from build123d import *

# Parameters (mm, degrees)
BOSS_EXTRUDE1_DEPTH   = 6
SKETCH2_W             = 71
SKETCH2_H             = 6
BOSS_EXTRUDE2_DEPTH   = 6
CUT_EXTRUDE1_DEPTH    = 6
SKETCH5_W             = 30
SKETCH5_H             = 6
BOSS_EXTRUDE3_DEPTH   = 6
BOSS_EXTRUDE3_2_DEPTH = 6
BOSS_EXTRUDE3_3_DEPTH = 6
BOSS_EXTRUDE3_4_DEPTH = 6


with BuildPart() as part:
    # Sketch1 → Boss-Extrude1 (new body)
    with BuildSketch(Plane(origin=(0, 0, 0), x_dir=(1, 0, 0), z_dir=(0, 1, 0))):
        Polygon((200, 469.3), (140.436469322, 469.3), (0, 0), (200, 0), align=None)
    extrude(amount=BOSS_EXTRUDE1_DEPTH)

    # Sketch2 → Boss-Extrude2 (add)
    with BuildSketch(Plane(origin=(200, 0, 0), x_dir=(0, 0, -1), z_dir=(1, 0, 0))):
        with Locations((402.4, 3)):
            Rectangle(SKETCH2_W, SKETCH2_H)
        with Locations((252.2, 3)):
            Rectangle(SKETCH2_W, SKETCH2_H)
        with Locations((102, 3)):
            Rectangle(SKETCH2_W, SKETCH2_H)
    extrude(amount=BOSS_EXTRUDE2_DEPTH)

    # Sketch4 → Cut-Extrude1 (cut)
    with BuildSketch(Plane(origin=(0, 6, 0), x_dir=(1, 0, 0), z_dir=(0, 1, 0))):
        Polygon((123.445854535, 355.88111854), (117.889311346, 357.54389567), (103.612362884, 309.834266216), (109.168906073, 308.171489086), align=None)
        Polygon((56.132049338, 130.936921838), (50.575506148, 132.599698968), (64.85245461, 180.309328422), (70.4089978, 178.646551292), align=None)
    extrude(amount=-CUT_EXTRUDE1_DEPTH, mode=Mode.SUBTRACT)


with BuildPart() as body_2:
    # Sketch5 → Boss-Extrude3 (new body)
    with BuildSketch(Plane.XZ):
        with Locations((160, 3)):
            Rectangle(SKETCH5_W, SKETCH5_H)
    extrude(amount=-BOSS_EXTRUDE3_DEPTH)


with BuildPart() as body_3:
    # Sketch5 → Boss-Extrude3 2 (new body)
    with BuildSketch(Plane.XZ):
        with Locations((120, 3)):
            Rectangle(SKETCH5_W, SKETCH5_H)
    extrude(amount=-BOSS_EXTRUDE3_2_DEPTH)


with BuildPart() as body_4:
    # Sketch5 → Boss-Extrude3 3 (new body)
    with BuildSketch(Plane.XZ):
        with Locations((80, 3)):
            Rectangle(SKETCH5_W, SKETCH5_H)
    extrude(amount=-BOSS_EXTRUDE3_3_DEPTH)


with BuildPart() as body_5:
    # Sketch5 → Boss-Extrude3 4 (new body)
    with BuildSketch(Plane.XZ):
        with Locations((40, 3)):
            Rectangle(SKETCH5_W, SKETCH5_H)
    extrude(amount=-BOSS_EXTRUDE3_4_DEPTH)


with BuildPart() as body_3_1:
    add(body_3.part)

    # Combine1: union body 2, body 4, body 5, part
    add(body_2.part)
    add(body_4.part)
    add(body_5.part)
    add(part.part)


solid = body_3_1.part
Source: CAD feature listing. Evaluate the final solid. Frame: model axes, mm. A direction names the side the tool comes from. Coordinates: 2 decimals unless noted, no trailing zeros. Loops run counter-clockwise (first coordinate to the right, second up) from the corner with the lowest first, then second, coordinate; pieces in that order, holes last. Notation, with made-up numbers: (-29.75, -37) -> (0.25, -37) arc R23 cw to (0.25, -3) -> close; hole circle Ø9 at (82.5, -7.5). An arc over 180 degrees is marked (long way). Answer in a Markdown table with one row per item. Add a question column.
Q1. Ray query, line 1 along Z through (x, y) = (179, 5.1); line 2 along X through (y, z) = (5.1, -343.5); line 3 along X through (y, z) = (3.65, -164). Return the intervals inside material, ascending.
Q2. Contact query for flat-ended pins moving along their axis: pin 1 Ø1 at (y, z) = (4.5, -335.5) entering from -X; pin 2 Ø3 at (x, y) = (203, 2) entering from +Z; pin 3 Ø3 at (y, z) = (3, 4) entering from +X. Output: stop coordinate, or through.
Q3. Pull-direction query (X, two-part tool) for faces 1 (the face through (57.614, 3.042, -156.121)), 2 (the face through (124, 0, -182)), 3 (the face through (71.201, 2.958, -237.935)); classes: pulls with the +X half, pulls with the -X half, needs draft (parallel to the pull), parting line crosses it, or undercut.
Q4. Section B-B on y = 0.9. Give the number of separate pieces and of enclosed holes in the cut face, and give its area (3 significant figures).
Q5. Section A-A on z = -150. Return the cut outline in (x, y), and give its area (3 significant figures).
Q6. Section C-C on z = -225. Return the cut outline in (x, y).
Q7. Reachability of faces 4 (the face through (110.85, 3.04, -334.02)), 5 (the face through (124, 6, -182)) from +Z, -Z, +X, -X, +Y, -Y: full face, straight path, thin tool, end or side. Return the list, or none.
Q8. Section D-D on x = 128. Return the cut outline in (y, z).
Computed values:
| question | item | result |
|---|---|---|
| 1 | line 1 | z = -469.3 to 0 |
| 1 | line 2 | x = 102.79 to 113.69, 119.74 to 200 |
| 1 | line 3 | x = 49.08 to 59.97, 66.03 to 200 |
| 2 | pin 1 | stops at x = 100.25 |
| 2 | pin 2 | stops at z = -66.5 |
| 2 | pin 3 | stops at x = 175 |
| 3 | face 1 | undercut |
| 3 | face 2 | needs draft |
| 3 | face 3 | pulls with the -X half |
| 4 | separate pieces | 1 |
| 4 | enclosed holes | 2 |
| 4 | area | 62,300 mm^2 |
| 5 | outline | (44.89, 0) -> (55.78, 0) -> (55.78, 6) -> (44.89, 6) -> close; (61.84, 0) -> (200, 0) -> (200, 6) -> (61.84, 6) -> close |
| 5 | area | 894 mm^2 |
| 6 | outline | (67.33, 0) -> (206, 0) -> (206, 6) -> (67.33, 6) -> close |
| 7 | face 4 | +Y, -Y |
| 7 | face 5 | +Z, -Z, +X, -X, +Y |
| 8 | outline | (0, -427.74) -> (6, -427.74) -> (6, 6) -> (0, 6) -> close |
